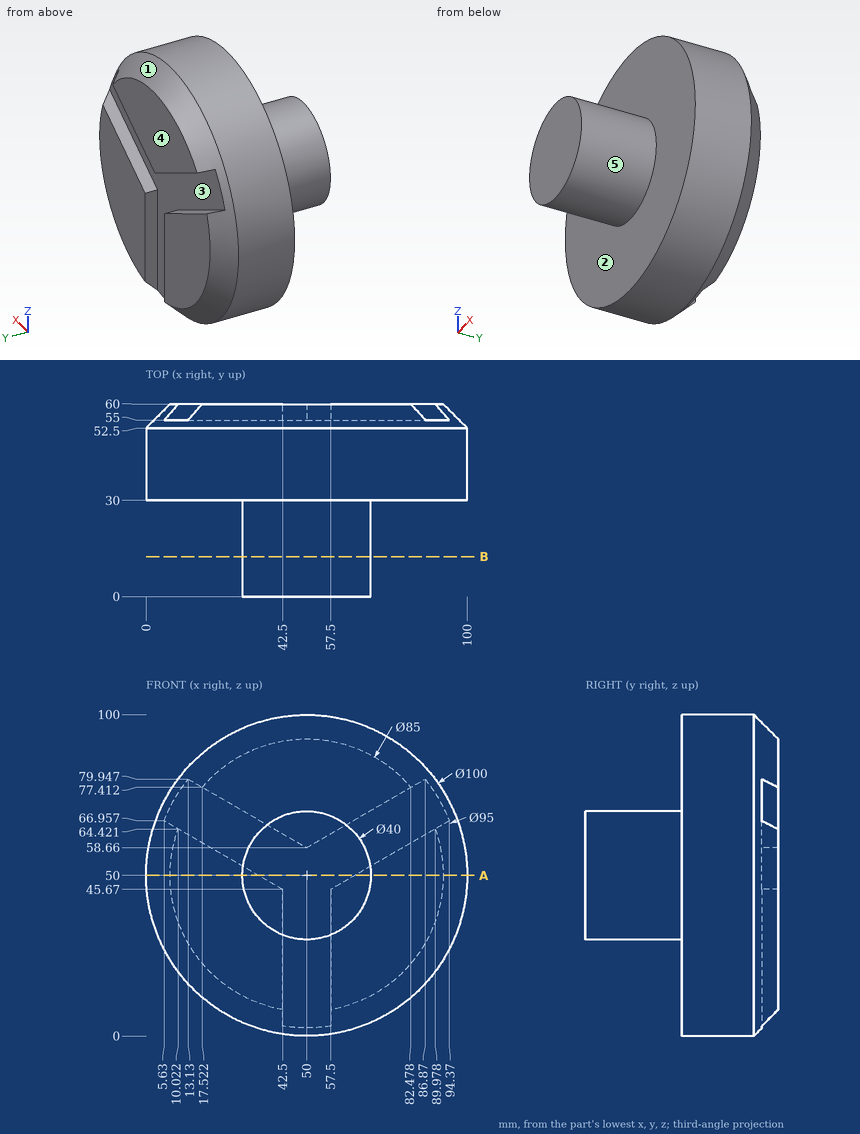
For this review, use the dimensioned drawing (mm, ordinates from the lowest corner) and the shaded views. A direction names the side the tool comes from. Round coordinates to 2 decimals unless told otherwise and drop trailing zeros. Loops run counter-clockwise (first coordinate to the right, second up) from the corner with the lowest first, then second, coordinate; pieces in that order, holes last. Notation, with made-up numbers: M 2,-30.5 L 59,-30.5 A25 ccw 59,-2.5 Z; hole C 86,-12 d7. An arc over 180 degrees is marked long. Answer as a JSON object with one key per item and string values.
(1) Take a section at B-B on y = 12.5. Give the boundary of the cut face in (x, z), and give its area (3 significant figures).
Resolved:
{"outline": "C 50,50 d40", "area": "1,260 mm²"}
(2) To check wall thickness, follow line 1 along Y through (x, z) = (38, 22.5); line 2 along Y through (x, z) = (77, 66.5); line 3 along Z through (x, y) = (49.5, 4). State the ranges of each line that lie inside material, in increasing order.
Resolved:
{"line 1": "30 to 60", "line 2": "30 to 55", "line 3": "30.01 to 69.99"}
(3) Tool access review of the marked faces 1 and 2: name each direction out of +Z, -Z, +X, -X, +Y, -Y from which nothing blocks a thin tool from reaching the whole face with its end or side.
Resolved:
{"face 1": "+Y", "face 2": "-Y"}
(4) Clearance check with flat-ended pins moving along their axes: P1, Ø5, axis at x = 47, y = 12, coming from the +Z side; P2, Ø12, axis at x = 12, y = 20, coming from the -Z side; P3, Ø2, axis at y = 42, z = 63, coming from the -X side; P4, Ø1.5, axis at y = 32.5, z = 27, coming from the -X side. State where each tip first meets the part, or that it passes through.
Resolved:
{"P1": "z = 69.99", "P2": "through", "P3": "x = 1.46", "P4": "x = 5.22"}
(5) Draft analysis for pull direction Z (two halves, no side actions). For the marked faces 3, 4 and 5, state which applies: released by +Z, released by -Z, zero draft, split by the parting line, or undercut.
Resolved:
{"face 3": "undercut", "face 4": "zero draft", "face 5": "split by the parting line"}
(6) Take a section at A-A on z = 50. Give the boundary of the cut face in (x, y).
Resolved:
{"outline": "M 0,30 L 30,30 L 30,0 L 70,0 L 70,30 L 100,30 L 100,52.5 L 92.5,60 L 65,60 L 65,55 L 35,55 L 35,60 L 7.5,60 L 0,52.5 Z"}
